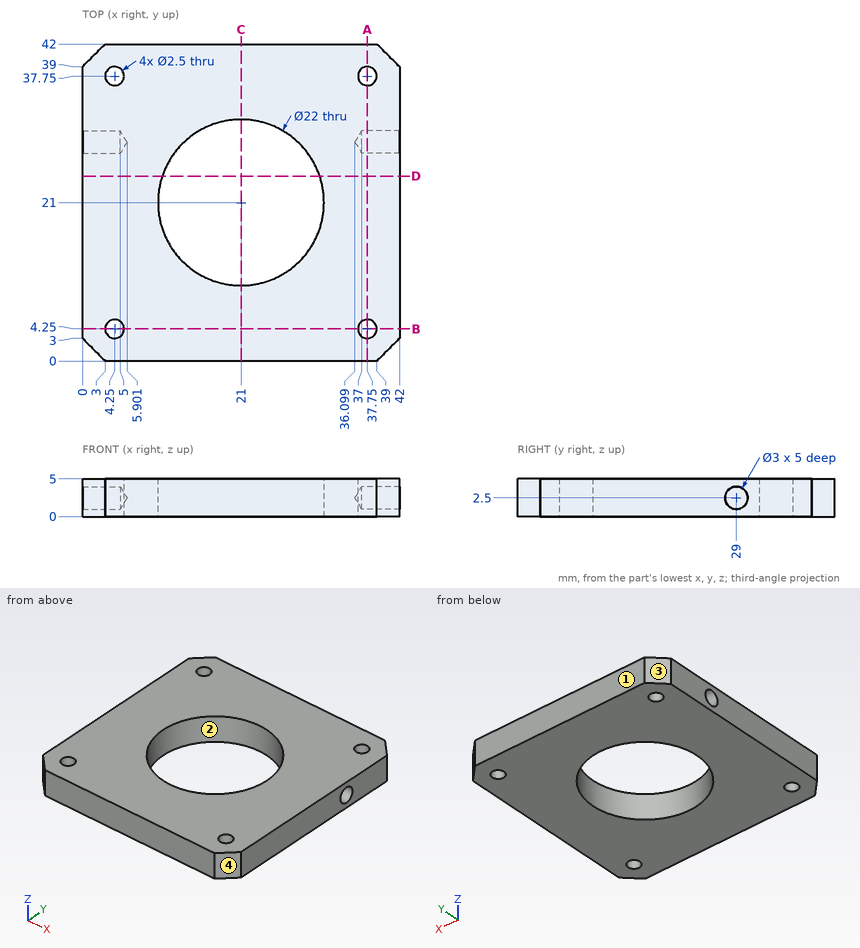
Input: dimensioned drawing with shaded views. Units: mm. Origin: part minimum x, y, z. Coordinates: 2 decimals unless noted, no trailing zeros. Write each loop counter-clockwise with the first axis right and the second up, starting at its lowest first coordinate (ties: lowest second). Pieces come first, ordered by that corner, then holes. Notation, with made-up numbers: (80.5, -17) -> (89.5, -17) arc R4 cw to (89.5, -11) -> close; hole circle Ø1 at (85, -28). An arc over 180 degrees is marked (long way). Return JSON: item names as keys, results as strings. Group by question number.
1) Section query A-A, the plane x = 37.75. Return loops of the section in (y, z), plus the area to 3 significant figures.
2) Mould query, pull axis X, two halves, no side actions, for the marked faces 1, 2, 3 and 4. Classes: +X half, -X half, draft (parallel to the pull), parting line (faces both ways), or undercut.
3) Section query C-C, the plane x = 21. Return loops of the section in (y, z).
4) Ray query, line 1 along Y through (x, z) = (20.5, 4.85); line 2 along Z through (x, y) = (2, 29); line 3 along Y through (x, z) = (40.5, 2.4) (1 decimal). Return the intervals inside material, ascending.
5) Section query D-D, the plane y = 24.5. Return loops of the section in (x, z), plus the area to 3 significant figures.
6) Contact query for a flat-ended pin moving along its axis: P1, Ø3, axis at x = 28.5, y = 19.5, coming from the +Z side. Output: stop coordinate, or through.
7) Section query B-B, the plane y = 4.25. Return loops of the section in (x, z), plus the area to 3 significant figures.
From the geometry:
{
 "1": {"outline": "(0, 0) -> (3, 0) -> (3, 5) -> (0, 5) -> close; (5.5, 0) -> (36.5, 0) -> (36.5, 5) -> (5.5, 5) -> close; (39, 0) -> (42, 0) -> (42, 5) -> (39, 5) -> close; hole circle Ø3 at (29, 2.5)", "area": "178 mm²"},
 "2": {"face 1": "draft", "face 2": "undercut", "face 3": "-X half", "face 4": "+X half"},
 "3": {"outline": "(0, 0) -> (10, 0) -> (10, 5) -> (0, 5) -> close; (32, 0) -> (42, 0) -> (42, 5) -> (32, 5) -> close"},
 "4": {"line 1": "0 to 10.01, 31.99 to 42", "line 2": "0 to 1, 4 to 5", "line 3": "1.5 to 27.5, 30.5 to 40.5"},
 "5": {"outline": "(0, 0) -> (10.57, 0) -> (10.57, 5) -> (0, 5) -> close; (31.43, 0) -> (42, 0) -> (42, 5) -> (31.43, 5) -> close", "area": "106 mm²"},
 "6": {"P1": "through"},
 "7": {"outline": "(0, 0) -> (3, 0) -> (3, 5) -> (0, 5) -> close; (5.5, 0) -> (36.5, 0) -> (36.5, 5) -> (5.5, 5) -> close; (39, 0) -> (42, 0) -> (42, 5) -> (39, 5) -> close", "area": "185 mm²"}
}
